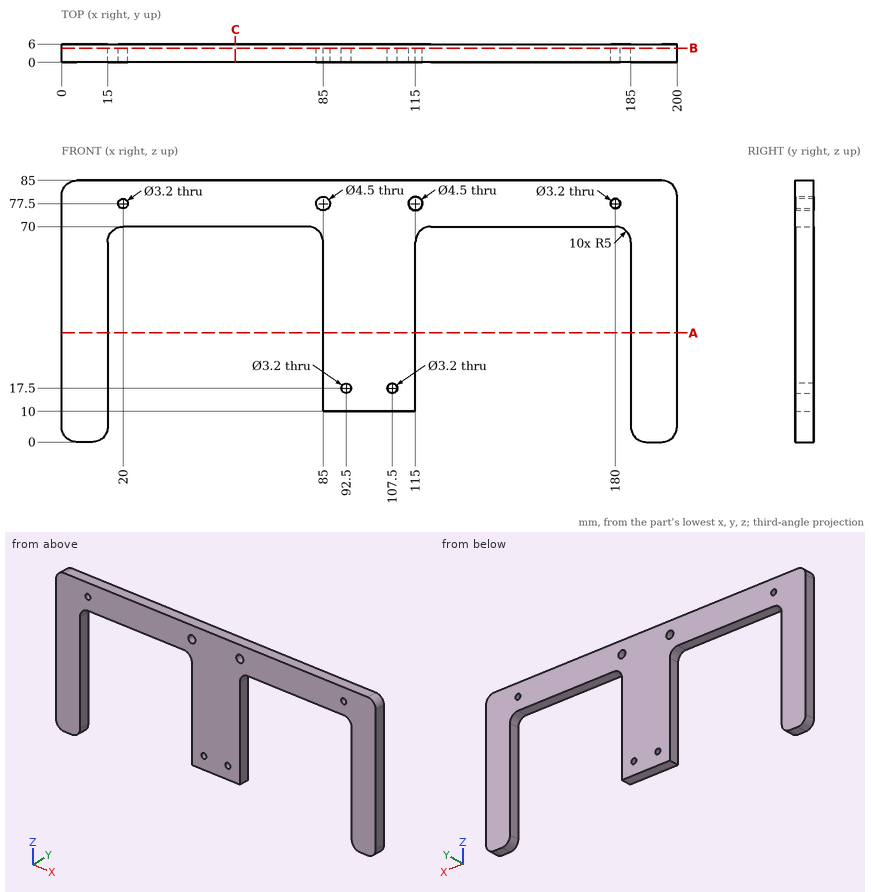
Source: three-view drawing plus pictorial views. Frame: mm from the lowest corner of the part. Coordinates: 2 decimals unless noted, no trailing zeros. Order: outer loops, then holes, each group sorted by start corner. A loop starts at its lowest first (then second) coordinate and runs counter-clockwise, first axis right, second up. Notation, with made-up numbers: (38.25, 23.25) -> (82.25, 23.25) arc R24 ccw to (82.25, 62.25) -> close; hole circle Ø11 at (77, 3). An arc over 180 degrees is marked (long way). Write item = value, one per line.
(1) Line query: line 1 (X direction, y = 0.45, z = 49.5); line 2 (X direction, y = 3.25, z = 17.5); line 3 (X direction, y = 2, z = 77.5). Output: solid intervals per line, ascending.
Solved:
line_1 = 0 to 15, 85 to 115, 185 to 200
line_2 = 0 to 15, 85 to 90.9, 94.1 to 105.9, 109.1 to 115, 185 to 200
line_3 = 0 to 18.4, 21.6 to 82.75, 87.25 to 112.75, 117.25 to 178.4, 181.6 to 200
(2) Pin query (flat end, axial travel): pin 1 Ø3 at (x, y) = (107, 4) entering from -Z; pin 2 Ø3 at (x, y) = (60.5, 4) entering from -Z. Return the tip coordinate at first contact, or that it passes through.
Solved:
pin_1 = 10
pin_2 = 70
(3) Cut plane A-A on z = 35.5. Return loops of the section in (x, y), plus the area to 3 significant figures.
Solved:
outline = (0, 0) -> (15, 0) -> (15, 6) -> (0, 6) -> close; (85, 0) -> (115, 0) -> (115, 6) -> (85, 6) -> close; (185, 0) -> (200, 0) -> (200, 6) -> (185, 6) -> close
area = 360 mm²
(4) Cut plane B-B on y = 4.65. Return loops of the section in (x, z).
Solved:
outline = (0, 5) arc R5 ccw to (5, 0) -> (10, 0) arc R5 ccw to (15, 5) -> (15, 65) arc R5 cw to (20, 70) -> (80, 70) arc R5 cw to (85, 65) -> (85, 10) -> (115, 10) -> (115, 65) arc R5 cw to (120, 70) -> (180, 70) arc R5 cw to (185, 65) -> (185, 5) arc R5 ccw to (190, 0) -> (195, 0) arc R5 ccw to (200, 5) -> (200, 80) arc R5 ccw to (195, 85) -> (5, 85) arc R5 ccw to (0, 80) -> close; hole circle Ø3.2 at (20, 77.5); hole circle Ø4.5 at (85, 77.5); hole circle Ø3.2 at (92.5, 17.5); hole circle Ø3.2 at (107.5, 17.5); hole circle Ø4.5 at (115, 77.5); hole circle Ø3.2 at (180, 77.5)
(5) Cut plane C-C on x = 56.5. Return loops of the section in (y, z), plus the area to 3 significant figures.
Solved:
outline = (0, 70) -> (6, 70) -> (6, 85) -> (0, 85) -> close
area = 90.0 mm²
